```python
from build123d import *

# Parameters (mm, degrees)
ESQUISSE1_R      = 4
EXTRUSION1_DEPTH = 10


with BuildPart() as part:
    # Esquisse1 → Extrusion1 (new body)
    with BuildSketch(Plane.XY):
        with BuildLine():
            Line((4.000854566, 5.506703891), (4.118719306, 5.668930788))
            ThreePointArc((4.118719306, 5.668930788), (4.204956471, 6.058576718), (3.97856745, 6.387223657))
            ThreePointArc((3.97856745, 6.387223657), (3.416278511, 6.704824095), (2.828829213, 6.973044549))
            ThreePointArc((2.828829213, 6.973044549), (2.429880127, 6.96302329), (2.165338881, 6.664227827))
            Line((2.165338881, 6.664227827), (2.10337372, 6.473518672))
            ThreePointArc((2.10337372, 6.473518672), (1.871017944, 6.191143724), (1.508589384, 6.142457413))
            ThreePointArc((1.508589384, 6.142457413), (0.989447991, 6.247128754), (0.463369963, 6.308003906))
            ThreePointArc((0.463369963, 6.308003906), (0.133724818, 6.466303924), (0, 6.806660341))
            Line((0, 6.806660341), (0, 7.007183814))
            ThreePointArc((0, 7.007183814), (-0.159260799, 7.373102927), (-0.535587189, 7.505915758))
            ThreePointArc((-0.535587189, 7.505915758), (-1.177169349, 7.432354763), (-1.810081842, 7.304055635))
            ThreePointArc((-1.810081842, 7.304055635), (-2.126948085, 7.061451877), (-2.165338881, 6.664227827))
            Line((-2.165338881, 6.664227827), (-2.10337372, 6.473518672))
            ThreePointArc((-2.10337372, 6.473518672), (-2.125377663, 6.108497242), (-2.389971431, 5.856079026))
            ThreePointArc((-2.389971431, 5.856079026), (-2.871489911, 5.635616265), (-3.332877492, 5.375644391))
            ThreePointArc((-3.332877492, 5.375644391), (-3.692612433, 5.309951241), (-4.000854566, 5.506703891))
            Line((-4.000854566, 5.506703891), (-4.118719306, 5.668930788))
            ThreePointArc((-4.118719306, 5.668930788), (-4.462645857, 5.87135442), (-4.845165725, 5.757603156))
            ThreePointArc((-4.845165725, 5.757603156), (-5.320978528, 5.320978528), (-5.757603156, 4.845165725))
            ThreePointArc((-5.757603156, 4.845165725), (-5.87135442, 4.462645857), (-5.668930788, 4.118719306))
            Line((-5.668930788, 4.118719306), (-5.506703891, 4.000854566))
            ThreePointArc((-5.506703891, 4.000854566), (-5.309951241, 3.692612433), (-5.375644391, 3.332877492))
            ThreePointArc((-5.375644391, 3.332877492), (-5.635616265, 2.871489911), (-5.856079026, 2.389971431))
            ThreePointArc((-5.856079026, 2.389971431), (-6.108497242, 2.125377663), (-6.473518672, 2.10337372))
            Line((-6.473518672, 2.10337372), (-6.664227827, 2.165338881))
            ThreePointArc((-6.664227827, 2.165338881), (-7.061451877, 2.126948085), (-7.304055635, 1.810081842))
            ThreePointArc((-7.304055635, 1.810081842), (-7.432354763, 1.177169349), (-7.505915758, 0.535587189))
            ThreePointArc((-7.505915758, 0.535587189), (-7.373102927, 0.159260799), (-7.007183814, 0))
            Line((-7.007183814, 0), (-6.806660341, 0))
            ThreePointArc((-6.806660341, 0), (-6.466303924, -0.133724818), (-6.308003906, -0.463369963))
            ThreePointArc((-6.308003906, -0.463369963), (-6.247128754, -0.989447991), (-6.142457413, -1.508589384))
            ThreePointArc((-6.142457413, -1.508589384), (-6.191143724, -1.871017944), (-6.473518672, -2.10337372))
            Line((-6.473518672, -2.10337372), (-6.664227827, -2.165338881))
            ThreePointArc((-6.664227827, -2.165338881), (-6.96302329, -2.429880127), (-6.973044549, -2.828829213))
            ThreePointArc((-6.973044549, -2.828829213), (-6.704824095, -3.416278511), (-6.387223657, -3.97856745))
            ThreePointArc((-6.387223657, -3.97856745), (-6.058576718, -4.204956471), (-5.668930788, -4.118719306))
            Line((-5.668930788, -4.118719306), (-5.506703891, -4.000854566))
            ThreePointArc((-5.506703891, -4.000854566), (-5.152748289, -3.908983733), (-4.83092033, -4.082625842))
            ThreePointArc((-4.83092033, -4.082625842), (-4.472450391, -4.472450391), (-4.082625842, -4.83092033))
            ThreePointArc((-4.082625842, -4.83092033), (-3.908983733, -5.152748289), (-4.000854566, -5.506703891))
            Line((-4.000854566, -5.506703891), (-4.118719306, -5.668930788))
            ThreePointArc((-4.118719306, -5.668930788), (-4.204956471, -6.058576718), (-3.97856745, -6.387223657))
            ThreePointArc((-3.97856745, -6.387223657), (-3.416278511, -6.704824095), (-2.828829213, -6.973044549))
            ThreePointArc((-2.828829213, -6.973044549), (-2.429880127, -6.96302329), (-2.165338881, -6.664227827))
            Line((-2.165338881, -6.664227827), (-2.10337372, -6.473518672))
            ThreePointArc((-2.10337372, -6.473518672), (-1.871017944, -6.191143724), (-1.508589384, -6.142457413))
            ThreePointArc((-1.508589384, -6.142457413), (-0.989447991, -6.247128754), (-0.463369963, -6.308003906))
            ThreePointArc((-0.463369963, -6.308003906), (-0.133724818, -6.466303924), (0, -6.806660341))
            Line((0, -6.806660341), (0, -7.007183814))
            ThreePointArc((0, -7.007183814), (0.159260799, -7.373102927), (0.535587189, -7.505915758))
            ThreePointArc((0.535587189, -7.505915758), (1.177169349, -7.432354763), (1.810081842, -7.304055635))
            ThreePointArc((1.810081842, -7.304055635), (2.126948085, -7.061451877), (2.165338881, -6.664227827))
            Line((2.165338881, -6.664227827), (2.10337372, -6.473518672))
            ThreePointArc((2.10337372, -6.473518672), (2.125377663, -6.108497242), (2.389971431, -5.856079026))
            ThreePointArc((2.389971431, -5.856079026), (2.871489911, -5.635616265), (3.332877492, -5.375644391))
            ThreePointArc((3.332877492, -5.375644391), (3.692612433, -5.309951241), (4.000854566, -5.506703891))
            Line((4.000854566, -5.506703891), (4.118719306, -5.668930788))
            ThreePointArc((4.118719306, -5.668930788), (4.462645857, -5.87135442), (4.845165725, -5.757603156))
            ThreePointArc((4.845165725, -5.757603156), (5.320978528, -5.320978528), (5.757603156, -4.845165725))
            ThreePointArc((5.757603156, -4.845165725), (5.87135442, -4.462645857), (5.668930788, -4.118719306))
            Line((5.668930788, -4.118719306), (5.506703891, -4.000854566))
            ThreePointArc((5.506703891, -4.000854566), (5.309951241, -3.692612433), (5.375644391, -3.332877492))
            ThreePointArc((5.375644391, -3.332877492), (5.635616265, -2.871489911), (5.856079026, -2.389971431))
            ThreePointArc((5.856079026, -2.389971431), (6.108497242, -2.125377663), (6.473518672, -2.10337372))
            Line((6.473518672, -2.10337372), (6.664227827, -2.165338881))
            ThreePointArc((6.664227827, -2.165338881), (7.061451877, -2.126948085), (7.304055635, -1.810081842))
            ThreePointArc((7.304055635, -1.810081842), (7.432354763, -1.177169349), (7.505915758, -0.535587189))
            ThreePointArc((7.505915758, -0.535587189), (7.373102927, -0.159260799), (7.007183814, 0))
            Line((7.007183814, 0), (6.806660341, 0))
            ThreePointArc((6.806660341, 0), (6.466303924, 0.133724818), (6.308003906, 0.463369963))
            ThreePointArc((6.308003906, 0.463369963), (6.247128754, 0.989447991), (6.142457413, 1.508589384))
            ThreePointArc((6.142457413, 1.508589384), (6.191143724, 1.871017944), (6.473518672, 2.10337372))
            Line((6.473518672, 2.10337372), (6.664227827, 2.165338881))
            ThreePointArc((6.664227827, 2.165338881), (6.96302329, 2.429880127), (6.973044549, 2.828829213))
            ThreePointArc((6.973044549, 2.828829213), (6.704824095, 3.416278511), (6.387223657, 3.97856745))
            ThreePointArc((6.387223657, 3.97856745), (6.058576718, 4.204956471), (5.668930788, 4.118719306))
            Line((5.668930788, 4.118719306), (5.506703891, 4.000854566))
            ThreePointArc((5.506703891, 4.000854566), (5.152748289, 3.908983733), (4.83092033, 4.082625842))
            ThreePointArc((4.83092033, 4.082625842), (4.472450391, 4.472450391), (4.082625842, 4.83092033))
            ThreePointArc((4.082625842, 4.83092033), (3.908983733, 5.152748289), (4.000854566, 5.506703891))
        make_face()
        Circle(ESQUISSE1_R, mode=Mode.SUBTRACT)
    extrude(amount=EXTRUSION1_DEPTH)


solid = part.part
```
Work out the finished part from the listing and answer in its coordinate system (mm). A direction names the side the tool comes from. Round coordinates to 2 decimals unless told otherwise and drop trailing zeros. Write each question's results on one line, items separated by ' | '. Start each with the question number.
1. Find the intervals of material crossed by probe 1 along Y at (x, z) = (-2.5, 9); probe 2 along X at (y, z) = (-5.5, 5); probe 3 along X at (y, z) = (-3, 7.25), in increasing order. Write a range as from..to.
2. A tool of negligible diameter and unlimited length cuts with its end or side. For faces 4 (the face through (5.63, -2.88, 4.93)), 5 (the face through (0.997, 6.246, 4.93)), 6 (the face through (-0.997, -6.246, 4.93)), 7 (the face through (-5.63, 2.88, 4.93)), from which of +Z, -Z, +X, -X, +Y, -Y can it reach the whole face along a straight path? Write none if from no direction.
3. For a pull along X with two mould halves and no side action, classify faces 1 (the face through (-2.86, 5.64, 4.93)), 2 (the face through (7.43, -1.19, 4.93)), 3 (the face through (-3.424, -6.701, 4.93)) as +X half, -X half, draft (parallel to the pull), parting line (faces both ways), or undercut.
4. Given pin 1 Ø1.5 at (x, z) = (-3, 7.5) entering from +Y; pin 2 Ø1.5 at (y, z) = (4, 2) entering from +X; pin 3 Ø1 at (y, z) = (-1, 2) entering from -X, each flat-ended and moving along its own axis, determine where each tip first touches the part or whether it passes through.
Evaluation:
1) probe 1: y = -6.99..-3.12, 3.12..5.81 | probe 2: x = -4..3.12, 4..5.14 | probe 3: x = -6.9..-2.65, 2.65..5.57
2) face 4: +Z, -Z, +X | face 5: +Z, -Z, +Y | face 6: +Z, -Z, -Y | face 7: +Z, -Z, -X
3) face 1: undercut | face 2: +X half | face 3: -X half
4) pin 1: stops at y = 5.94 | pin 2: stops at x = 6.79 | pin 3: stops at x = -6.31
